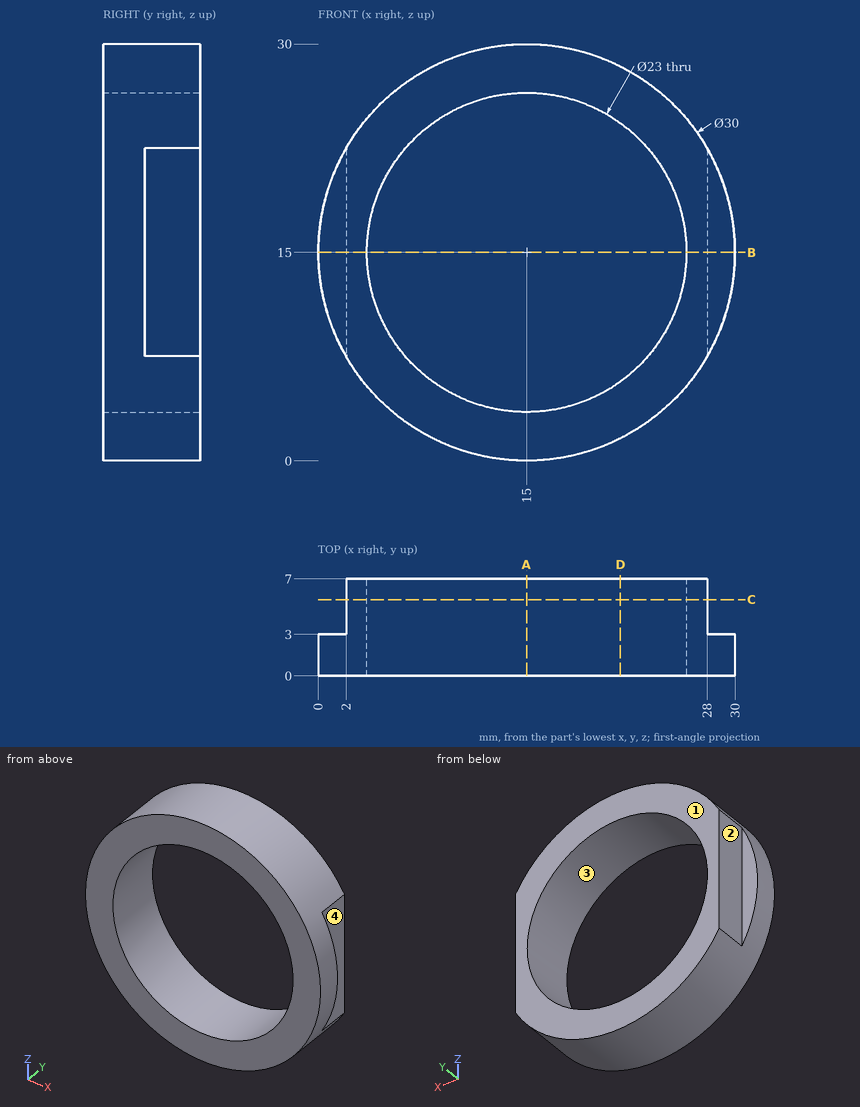
Input: dimensioned drawing with shaded views. Units: mm. Origin: part minimum x, y, z. Give positions to 0.01 mm unless a question says otherwise; leave off trailing zeros. Write each loop counter-clockwise with the first axis right and the second up, starting at its lowest first coordinate (ties: lowest second). Pieces come first, ordered by that corner, then holes.
1. Section query C-C, the plane y = 5.5. Return loops of the section in (x, z).
2. Pin query (flat end, axial travel): P1, Ø2, axis at x = 26.5, y = 3.5, coming from the +Z side; P2, Ø3, axis at y = 5, z = 14, coming from the -X side; P3, Ø10, axis at x = 3.5, z = 25, coming from the +Y side; P4, Ø3, axis at y = 4.5, z = 5.5, coming from the +X side. Return the tip coordinate at first contact, or that it passes through.
3. Draft query along X for the marked faces 1, 2, 3 and 4. Return one class per face: released by +X, released by -X, zero draft, split by the parting line, or undercut.
4. Section query A-A, the plane x = 15. Return loops of the section in (y, z), then the cut area to 3 significant figures.
5. Section query D-D, the plane x = 21.75. Return loops of the section in (y, z).
6. Section query B-B, the plane z = 15. Return loops of the section in (x, y), then the cut area to 3 significant figures.
7. Line query: probe 1 along Z at (x, y) = (15, 2.5); probe 2 along X at (y, z) = (5.25, 15). Output: solid intervals per line, ascending.
Computed:
1. outline: (2, 7.52) arc R15 ccw to (28, 7.52) - (28, 22.48) arc R15 ccw to (2, 22.48) - close; hole circle Ø23 at (15, 15)
2. P1: stops at z = 25.71
2. P2: stops at x = 2
2. P3: stops at y = 7
2. P4: stops at x = 27.69
3. face 1: zero draft
3. face 2: released by -X
3. face 3: undercut
3. face 4: released by +X
4. outline: (0, 0) - (7, 0) - (7, 3.5) - (0, 3.5) - close; (0, 26.5) - (7, 26.5) - (7, 30) - (0, 30) - close
4. area: 49.0 mm2
5. outline: (0, 1.6) - (7, 1.6) - (7, 5.69) - (0, 5.69) - close; (0, 24.31) - (7, 24.31) - (7, 28.4) - (0, 28.4) - close
6. outline: (0, 0) - (3.5, 0) - (3.5, 7) - (2, 7) - (2, 3) - (0, 3) - close; (26.5, 0) - (30, 0) - (30, 3) - (28, 3) - (28, 7) - (26.5, 7) - close
6. area: 33.0 mm2
7. probe 1: z = 0 to 3.5, 26.5 to 30
7. probe 2: x = 2 to 3.5, 26.5 to 28
